Model file for the job. Use its own axes, mm. Give positions to 0.01 mm unless a question says otherwise; leave off trailing zeros. Order: outer loops, then holes, each group sorted by start corner. A loop starts at its lowest first (then second) coordinate and runs counter-clockwise, first axis right, second up. Notation, with made-up numbers: M -29,11.25 L -21,11.25 A10 ccw -21,26.25 Z; hole C 81.25,14 d5. An arc over 180 degrees is marked long. Return JSON: item names as keys, results as strings. Group by question number.
1. Slice it at D-D on x = -12. List the corners of the cut face in (y, z) (1 decimal), then the cut area to 3 significant figures.
2. Slice it at A-A on y = -38.1. List the corners of the cut face in (x, z) (1 decimal), then the cut area to 3 significant figures.
3. Slice it at B-B on x = 0. List the corners of the cut face in (y, z) (1 decimal).
4. Wall check: probe 1 along Y at (x, z) = (0, -2); probe 2 along Y at (x, z) = (-10, 2); probe 3 along Y at (x, z) = (22, 2). Give the ranges that are in metal, low to high. Write a range as [from, to].
5. Pin check, flat tip, straight feed: pin 1 (4 mm diameter, centred on x = 0, y = 16.51, fed in from -Z). Stop position of the tip, or through.
6. Slice it at C-C on z = -1. Give the number of separate pieces and of enclosed holes in the cut face, then the cut area to 3 significant figures.
from build123d import *

# Parameters (mm, degrees)
SKETCH1_W             = 57.15
SKETCH1_H             = 136.525
SKETCH1_R             = 14.2875
BOSS_EXTRUDE1_DEPTH   = 3.175
F_8_CLEARANCE_HOLE1_D = 4.4958
F_8_CLEARANCE_HOLE2_D = 4.4958


with BuildPart() as part:
    # Sketch1 → Boss-Extrude1 (new, symmetric)
    with BuildSketch(Plane.XY):
        Rectangle(SKETCH1_W, SKETCH1_H)
        with Locations((0, 38.1)):
            Circle(SKETCH1_R, mode=Mode.SUBTRACT)
        with Locations((0, -38.1)):
            Circle(SKETCH1_R, mode=Mode.SUBTRACT)
    extrude(amount=BOSS_EXTRUDE1_DEPTH, both=True)

    # #8 Clearance Hole1 (through all)
    with Locations(Plane.XY.offset(3.175)):
        with Locations((0, -14.2875), (20.622229928, -26.19375), (20.622229928, -50.00625), (0, -61.9125), (-20.622229928, -50.00625), (-20.622229928, -26.19375), (0, -38.1)):
            Hole(F_8_CLEARANCE_HOLE1_D / 2)

    # #8 Clearance Hole2 (through all)
    with Locations(Plane.XY.offset(3.175)):
        with Locations((-12.7, 55.5625), (12.7, 55.5625), (0, 16.51)):
            Hole(F_8_CLEARANCE_HOLE2_D / 2)


solid = part.part
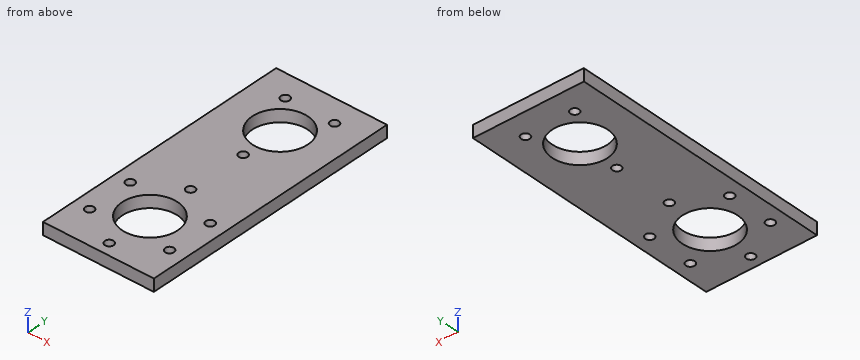
Result:
{
 "1": {"outline": "M -68.3,-3.2 L -45.9,-3.2 L -45.9,3.2 L -68.3,3.2 Z; M -30.3,-3.2 L 30.3,-3.2 L 30.3,3.2 L -30.3,3.2 Z; M 45.9,-3.2 L 53.4,-3.2 L 53.4,3.2 L 45.9,3.2 Z; M 57.7,-3.2 L 68.3,-3.2 L 68.3,3.2 L 57.7,3.2 Z", "area": "643 mm2"},
 "2": {"outline": "M -28.6,-3.2 L -14.3,-3.2 L -14.3,3.2 L -28.6,3.2 Z; M 14.3,-3.2 L 28.6,-3.2 L 28.6,3.2 L 14.3,3.2 Z", "area": "181 mm2"},
 "3": {"outline": "M -68.3,-3.2 L -64.2,-3.2 L -64.2,3.2 L -68.3,3.2 Z; M -59.7,-3.2 L -52.4,-3.2 L -52.4,3.2 L -59.7,3.2 Z; M -23.8,-3.2 L -16.5,-3.2 L -16.5,3.2 L -23.8,3.2 Z; M -12,-3.2 L 14.3,-3.2 L 14.3,3.2 L -12,3.2 Z; M 18.8,-3.2 L 23.8,-3.2 L 23.8,3.2 L 18.8,3.2 Z; M 52.4,-3.2 L 68.3,-3.2 L 68.3,3.2 L 52.4,3.2 Z"},
 "4": {"probe 1": "y = [-68.26, -64.16], [-59.66, -52.39], [-23.81, -16.54], [-12.04, 14.26], [18.76, 23.81], [52.39, 68.26]", "probe 2": "y = [-68.26, -48.3], [-27.9, 27.9], [48.3, 68.26]", "probe 3": "y = [-68.26, -51.78], [-48.23, -27.97], [-24.42, 68.26]"},
 "5": {"pin 1": "passes through"},
 "6": {"separate pieces": "1", "enclosed holes": "11", "area": "6,380 mm2"}
}
